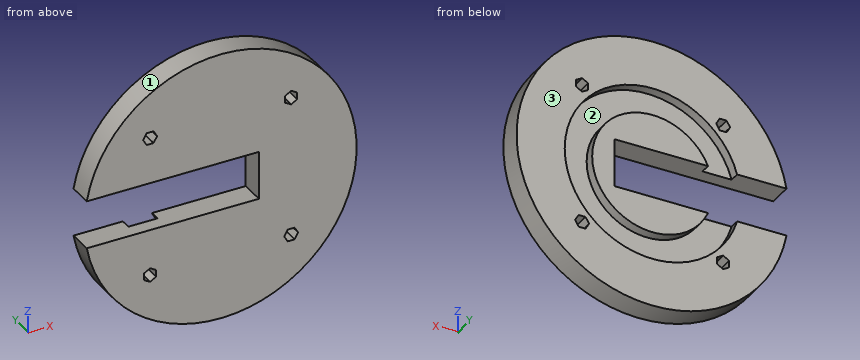
```python
from build123d import *

# Parameters (mm, degrees)
SKETCH_1_R          = 67.5
EXTRUDE_1_DEPTH     = 12
SKETCH_2_W          = 60
SKETCH_2_H          = 24
CUT_EXTRUDE_1_DEPTH = 97.210706265
CUT_EXTRUDE_3_DEPTH = 97.210706265
SKETCH_5_R          = 43.625
SKETCH_5_R_2        = 30
CUT_EXTRUDE_4_DEPTH = 5
SKETCH_6_W          = 75.06754016
SKETCH_6_H          = 24
CUT_EXTRUDE_5_DEPTH = 97.210706265


with BuildPart() as part:
    # 草图1 → 凸台-拉伸1 (new body)
    with BuildSketch(Plane(origin=(0, 0, 0), x_dir=(1, 0, 0), z_dir=(0, 1, 0))):
        with Locations(Location((0, 0, 0), (0, 0, 270))):
            Circle(SKETCH_1_R)
    extrude(amount=EXTRUDE_1_DEPTH)

    # 草图2 → 切除-拉伸1 (cut, through all)
    with BuildSketch(Plane(origin=(0, 12, 0), x_dir=(1, 0, 0), z_dir=(0, 1, 0))):
        with Locations((-11, 0)):
            Rectangle(SKETCH_2_W, SKETCH_2_H)
    extrude(amount=-CUT_EXTRUDE_1_DEPTH, mode=Mode.SUBTRACT)

    # 草图4 → 切除-拉伸3 (cut, through all)
    with BuildSketch(Plane(origin=(0, 12, 0), x_dir=(1, 0, 0), z_dir=(0, 1, 0))):
        Polygon((35.001785669, -38.465887284), (38.001785669, -36.733836476), (38.001785669, -33.269734861), (35.001785669, -31.537684054), (32.001785669, -33.269734861), (32.001785669, -36.733836476), align=None)
        Polygon((38.465887284, 35.001785669), (36.733836476, 38.001785669), (33.269734861, 38.001785669), (31.537684054, 35.001785669), (33.269734861, 32.001785669), (36.733836476, 32.001785669), align=None)
        Polygon((-38.465887284, -35.001785669), (-36.733836476, -38.001785669), (-33.269734861, -38.001785669), (-31.537684054, -35.001785669), (-33.269734861, -32.001785669), (-36.733836476, -32.001785669), align=None)
        Polygon((-35.001785669, 38.465887284), (-38.001785669, 36.733836476), (-38.001785669, 33.269734861), (-35.001785669, 31.537684054), (-32.001785669, 33.269734861), (-32.001785669, 36.733836476), align=None)
    extrude(amount=-CUT_EXTRUDE_3_DEPTH, mode=Mode.SUBTRACT)

    # 草图5 → 切除-拉伸4 (cut)
    with BuildSketch(Plane(origin=(0, 12, 0), x_dir=(1, 0, 0), z_dir=(0, 1, 0))):
        with Locations(Location((0, 0, 0), (0, 0, 270))):
            Circle(SKETCH_5_R)
        Circle(SKETCH_5_R_2, mode=Mode.SUBTRACT)
    extrude(amount=-CUT_EXTRUDE_4_DEPTH, mode=Mode.SUBTRACT)

    # 草图6 → 切除-拉伸5 (cut, through all)
    with BuildSketch(Plane(origin=(0, 12, 0), x_dir=(1, 0, 0), z_dir=(0, 1, 0))):
        with Locations((-78.53377008, 0)):
            Rectangle(SKETCH_6_W, SKETCH_6_H)
    extrude(amount=-CUT_EXTRUDE_5_DEPTH, mode=Mode.SUBTRACT)


solid = part.part
```
Geometry check sheet. Reference: the model listing, model coordinates, mm. Face numbers are marked on the shaded views. Give positions to 0.01 mm unless a question says otherwise; leave off trailing zeros. Order: outer loops, then holes, each group sorted by start corner. A loop starts at its lowest first (then second) coordinate and runs counter-clockwise, first axis right, second up. Notation, with made-up numbers: (-16.5, -33) - (30.5, -33) arc R33 cw to (30.5, -4) - close; hole circle Ø4 at (59.5, -16). An arc over 180 degrees is marked (long way). Answer in a Markdown table with one row per item. Add a question column.
Q1. Material ranges on probe 1 along Z at (x, y) = (0, 8.9) (3 decimals); probe 2 along Z at (x, y) = (33.5, 4); probe 3 along Z at (x, y) = (-33.5, 10.5), recorded low to high. Write a range as from..to.
Q2. Cross-section at C-C, the plane z = 0. Enter the section's corners in (x, y) (3 decimals).
Q3. Cross-section at B-B, the plane y = 5. Enter the section's corners in (x, z), then the cut area to 3 significant figures.
Q4. Mould release check, pull along X, two halves, no side actions. Record for the marked faces 1, 2 and 3: pulls with the +X half, pulls with the -X half, needs draft (parallel to the pull), parting line crosses it, or undercut.
Q5. Gauge pin test, flat ends, axial feed: pin 1 (4 mm diameter, centred on x = 35, y = 8, fed in from +Z); pin 2 (1.5 mm diameter, centred on x = 36, y = 4.5, fed in from -Z); pin 3 (1.7 mm diameter, centred on y = 4, z = -34.5, fed in from +X). Record the tip position at first contact, or that the pin passes through.
Q6. Cross-section at A-A, the plane x = 0. Enter the section's corners in (y, z) (3 decimals).
Q7. Cross-section at D-D, the plane x = 22.5. Enter the section's corners in (y, z) (3 decimals).
Check values:
| question | item | result |
|---|---|---|
| 1 | probe 1 | z = -67.5..-43.625, -30..-12, 12..30, 43.625..67.5 |
| 1 | probe 2 | z = -58.6..-38, -32..32.4, 37.6..58.6 |
| 1 | probe 3 | z = -58.6..-37.6, -32.4..-27.94, 27.94..32, 38..58.6 |
| 2 | outline | (19, 0) - (67.5, 0) - (67.5, 12) - (43.625, 12) - (43.625, 7) - (30, 7) - (30, 12) - (19, 12) - close |
| 3 | outline | (-66.42, -12) arc R67.5 ccw (long way) to (-66.42, 12) - (19, 12) - (19, -12) - close; hole (-38.47, 35) - (-36.73, 32) - (-33.27, 32) - (-31.54, 35) - (-33.27, 38) - (-36.73, 38) - close; hole (-38, -36.73) - (-35, -38.47) - (-32, -36.73) - (-32, -33.27) - (-35, -31.54) - (-38, -33.27) - close; hole (31.54, -35) - (33.27, -38) - (36.73, -38) - (38.47, -35) - (36.73, -32) - (33.27, -32) - close; hole (32, 33.27) - (35, 31.54) - (38, 33.27) - (38, 36.73) - (35, 38.47) - (32, 36.73) - close |
| 3 | area | 12,100 mm^2 |
| 4 | face 1 | parting line crosses it |
| 4 | face 2 | undercut |
| 4 | face 3 | needs draft |
| 5 | pin 1 | stops at z = 58.88 |
| 5 | pin 2 | stops at z = -57.56 |
| 5 | pin 3 | stops at x = 58.51 |
| 6 | outline | (0, -67.5) - (12, -67.5) - (12, -43.625) - (7, -43.625) - (7, -30) - (12, -30) - (12, -12) - (0, -12) - close; (0, 12) - (12, 12) - (12, 30) - (7, 30) - (7, 43.625) - (12, 43.625) - (12, 67.5) - (0, 67.5) - close |
| 7 | outline | (0, -63.64) - (12, -63.64) - (12, -37.375) - (7, -37.375) - (7, -19.843) - (12, -19.843) - (12, 19.843) - (7, 19.843) - (7, 37.375) - (12, 37.375) - (12, 63.64) - (0, 63.64) - close |
